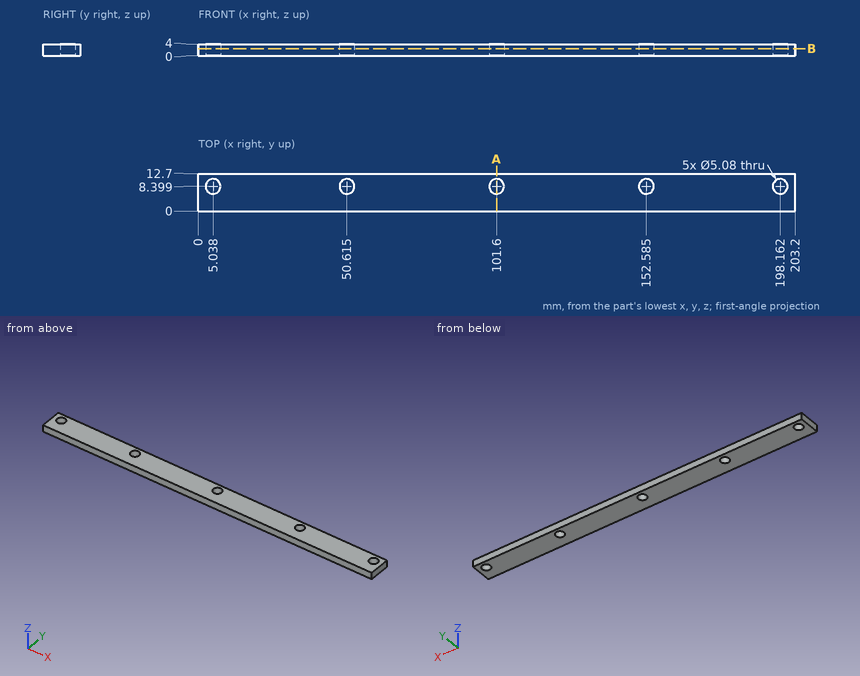
The figure shows three views and two pictorial views of one solid part (mm, origin at its lowest corner). Answer the questions. Give positions to 0.01 mm unless a question says otherwise; leave off trailing zeros. Order: outer loops, then holes, each group sorted by start corner. A loop starts at its lowest first (then second) coordinate and runs counter-clockwise, first axis right, second up. Notation, with made-up numbers: M -30.5,35.5 L 11.5,35.5 A22 ccw 11.5,57.5 Z; hole C 62,79.25 d4. An arc over 180 degrees is marked long. Return JSON: item names as keys, results as strings.
1) This flat-tipped pin is pushed along its axis until it touches: pin 1 (2 mm diameter, centred on x = 65, y = 10.5, fed in from -Z). Where does it stop, or does it pass through?
Resolved:
{"pin 1": "z = 0"}
2) Section B-B, the plane z = 2.45 is taken. Write down the section's boundary in (x, y) (1 decimal), plus the area to 3 significant figures.
Resolved:
{"outline": "M 0,0 L 203.2,0 L 203.2,12.7 L 0,12.7 Z; hole C 5,8.4 d5.1; hole C 50.6,8.4 d5.1; hole C 101.6,8.4 d5.1; hole C 152.6,8.4 d5.1; hole C 198.2,8.4 d5.1", "area": "2,480 mm^2"}
3) Straight lines are drawn through the part: line 1 along X through (y, z) = (8, 1.55); line 2 along Y through (x, z) = (101.6, 2.05); line 3 along X through (y, z) = (9, 3.55) (1 decimal). For each, find the intervals that lie inside material, in ascending order. Write a range as [from, to].
Resolved:
{"line 1": "[0, 2.53], [7.55, 48.11], [53.12, 99.09], [104.11, 150.08], [155.09, 195.65], [200.67, 203.2]", "line 2": "[0, 5.86], [10.94, 12.7]", "line 3": "[0, 2.6], [7.5, 48.1], [53.1, 99.1], [104.1, 150.1], [155.1, 195.7], [200.6, 203.2]"}
4) Section A-A, the plane x = 101.6 is taken. Write down the section's boundary in (y, z).
Resolved:
{"outline": "M 0,0 L 5.86,0 L 5.86,4 L 0,4 Z; M 10.94,0 L 12.7,0 L 12.7,4 L 10.94,4 Z"}
